Source: CAD feature listing. Evaluate the final solid. Frame: model axes, mm. Round coordinates to 2 decimals unless told otherwise and drop trailing zeros. Loops run counter-clockwise (first coordinate to the right, second up) from the corner with the lowest first, then second, coordinate; pieces in that order, holes last. Notation, with made-up numbers: (51.5, 48) -> (84.5, 48) arc R25 cw to (84.5, 74) -> close; hole circle Ø9 at (-1, 3.25). An arc over 180 degrees is marked (long way). Put each result on its own line as item: value. Start each with the question number.
1. Material intervals for L1, parallel to Z at x = 31.5, y = 2, sorted ascending.
2. Cut plane B-B (z = 0.25). Return the cut outline in (x, y), then the cut area to 3 significant figures.
3. Cut plane A-A (y = 4). Return the cut outline in (x, z) (3 decimals).
4. Contact query for a flat-ended pin moving along its axis: pin 1 (4 mm diameter, centred on x = -19.51, z = -0.2, fed in from +Y). Output: stop coordinate, or through.
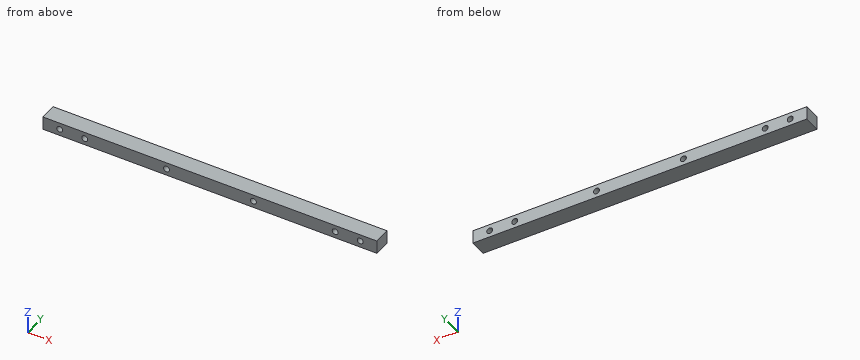
```python
from build123d import *

# Parameters (mm, degrees)
SKETCH1_W           = 200
SKETCH1_H           = 8
BOSS_EXTRUDE1_DEPTH = 10
SKETCH2_R           = 1.775
CUT_EXTRUDE1_DEPTH  = 108.045777637
SKETCH3_R           = 1.775
CUT_EXTRUDE2_DEPTH  = 108.045777637


with BuildPart() as part:
    # Sketch1 → Boss-Extrude1 (new body)
    with BuildSketch(Plane(origin=(0, 0, 0), x_dir=(1, 0, 0), z_dir=(0, 1, 0))):
        with Locations((6.494727973, 0.203739262)):
            Rectangle(SKETCH1_W, SKETCH1_H)
    extrude(amount=BOSS_EXTRUDE1_DEPTH)

    # Sketch2 → Cut-Extrude1 (cut, through all)
    with BuildSketch(Plane(origin=(0, 10, 0), x_dir=(1, 0, 0), z_dir=(0, 1, 0))):
        with Locations(Location((-19.505272027, 0.203739262, 0), (0, 0, 270))):
            Circle(SKETCH2_R)
        with Locations(Location((32.494727973, 0.203739262, 0), (0, 0, 270))):
            Circle(SKETCH2_R)
    extrude(amount=-CUT_EXTRUDE1_DEPTH, mode=Mode.SUBTRACT)

    # Sketch3 → Cut-Extrude2 (cut, through all)
    with BuildSketch(Plane(origin=(0, 10, 0), x_dir=(1, 0, 0), z_dir=(0, 1, 0))):
        with Locations(Location((-83.505272027, 0.203739262, 0), (0, 0, 270))):
            Circle(SKETCH3_R)
        with Locations(Location((-68.505272027, 0.203739262, 0), (0, 0, 270))):
            Circle(SKETCH3_R)
        with Locations(Location((81.494727973, 0.203739262, 0), (0, 0, 270))):
            Circle(SKETCH3_R)
        with Locations(Location((96.494727973, 0.203739262, 0), (0, 0, 270))):
            Circle(SKETCH3_R)
    extrude(amount=-CUT_EXTRUDE2_DEPTH, mode=Mode.SUBTRACT)


solid = part.part
```
Solution:
1. L1: z = -4.2 to -1.67, 1.27 to 3.8
2. outline: (-93.51, 0) -> (-85.22, 0) -> (-85.22, 10) -> (-93.51, 10) -> close; (-81.79, 0) -> (-70.22, 0) -> (-70.22, 10) -> (-81.79, 10) -> close; (-66.79, 0) -> (-21.22, 0) -> (-21.22, 10) -> (-66.79, 10) -> close; (-17.79, 0) -> (30.78, 0) -> (30.78, 10) -> (-17.79, 10) -> close; (34.21, 0) -> (79.78, 0) -> (79.78, 10) -> (34.21, 10) -> close; (83.21, 0) -> (94.78, 0) -> (94.78, 10) -> (83.21, 10) -> close; (98.21, 0) -> (106.49, 0) -> (106.49, 10) -> (98.21, 10) -> close
2. area: 1,790 mm^2
3. outline: (-93.505, -4.204) -> (106.495, -4.204) -> (106.495, 3.796) -> (-93.505, 3.796) -> close; hole circle Ø3.55 at (-83.505, -0.204); hole circle Ø3.55 at (-68.505, -0.204); hole circle Ø3.55 at (-19.505, -0.204); hole circle Ø3.55 at (32.495, -0.204); hole circle Ø3.55 at (81.495, -0.204); hole circle Ø3.55 at (96.495, -0.204)
4. pin 1: stops at y = 10
